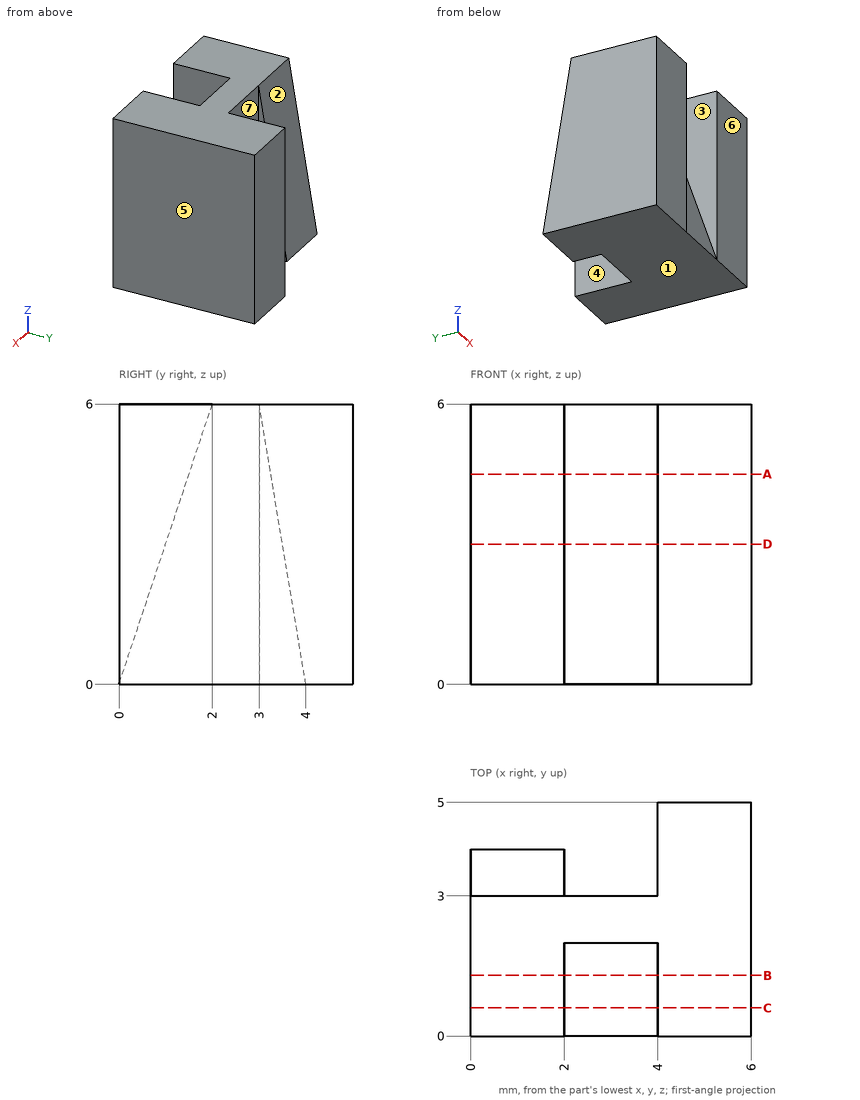
Study the drawing (mm; zero at the part's minimum x, y, z) and answer. A direction names the side the tool comes from. Coordinates: 2 decimals unless noted, no trailing zeros. Write each loop counter-clockwise with the first axis right and the second up, starting at its lowest first coordinate (ties: lowest second). Pieces come first, ordered by that corner, then holes.
Q1. Which of the six approach directions +Z, -Z, +X, -X, +Y, -Y give full straight-line access (tool end or side, diameter ignored) to the marked faces 1, 2, 3 and 4?
Q2. This flat-tipped pin is pushed along its axis until it touches: pin 1 Ø0.6 at (x, z) = (3.5, 4.5) entering from +Y. Where does it stop, or does it pass through?
Q3. A cutting plane is placed at A-A, the plane z = 4.5. Give the vertices of the cut face in (x, y), then the cut area to 3 significant figures.
Q4. A cutting plane is placed at B-B, the plane y = 1.3. Give the vertices of the cut face in (x, z).
Q5. A cutting plane is placed at D-D, the plane z = 3. Give the vertices of the cut face in (x, y), then the cut area to 3 significant figures.
Q6. A cutting plane is placed at C-C, the plane y = 0.6. Give the vertices of the cut face in (x, z), then the cut area to 3 significant figures.
Q7. Find the intervals of material crossed by line 1 (X direction, y = 0.55, z = 3.75); line 2 (X direction, y = 4.55, z = 0.5); line 3 (Y direction, x = 2.05, z = 1.75), in increasing order.
Q8. Determine the mould class of the marked faces 5, 6 and 7 for opening direction X: released by +X, released by -X, zero draft, split by the parting line, or undercut.
Findings below:
1. face 1: -Z, +X, -X, +Y, -Y
1. face 2: +Z, -X, +Y
1. face 3: +Z, -Y
1. face 4: +Z, -Z, +Y
2. pin 1: stops at y = 3
3. outline: (0, 0) - (2, 0) - (2, 1.5) - (4, 1.5) - (4, 0) - (6, 0) - (6, 5) - (4, 5) - (4, 3) - (2, 3) - (2, 3.25) - (0, 3.25) - close
3. area: 19.5 mm2
4. outline: (0, 0) - (6, 0) - (6, 6) - (4, 6) - (4, 3.9) - (2, 3.9) - (2, 6) - (0, 6) - close
5. outline: (0, 0) - (2, 0) - (2, 1) - (4, 1) - (4, 0) - (6, 0) - (6, 5) - (4, 5) - (4, 3) - (2, 3) - (2, 3.5) - (0, 3.5) - close
5. area: 21.0 mm2
6. outline: (0, 0) - (6, 0) - (6, 6) - (4, 6) - (4, 1.8) - (2, 1.8) - (2, 6) - (0, 6) - close
6. area: 27.6 mm2
7. line 1: x = 0 to 2, 4 to 6
7. line 2: x = 4 to 6
7. line 3: y = 0.58 to 3
8. face 5: released by +X
8. face 6: zero draft
8. face 7: undercut
